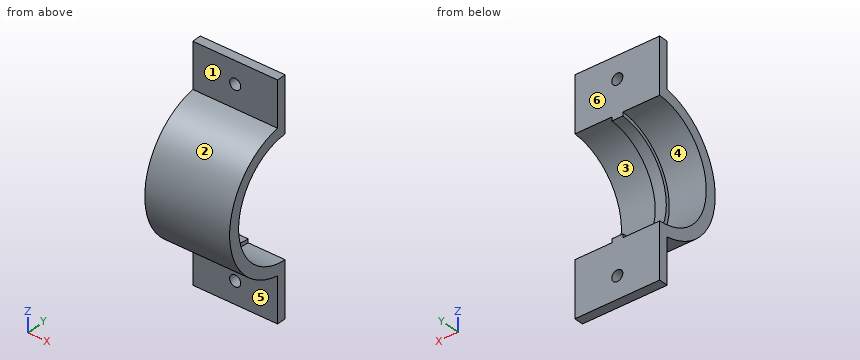
```python
from build123d import *

# Parameters (mm, degrees)
SKETCH3_W           = 13.566130208
SKETCH3_H           = 6
BOSS_EXTRUDE1_DEPTH = 11.5
SKETCH4_R           = 1.5
CUT_EXTRUDE1_DEPTH  = 11.5
SKETCH5_W           = 75.75040558
SKETCH5_H           = 1
CUT_EXTRUDE2_DEPTH  = 26


with BuildPart() as part:
    # Sketch2 → Revolve1 (revolve)
    with BuildSketch(Plane(origin=(0, 0, 0), x_dir=(1, 0, 0), z_dir=(0, 1, 0)), mode=Mode.PRIVATE) as revolve1_sk:
        Polygon((-11.5, 16), (-1.5, 16), (-1.5, 15), (1.5, 15), (1.5, 16), (11.5, 16), (11.5, 19), (-11.5, 19), align=None)
    revolve(revolve1_sk.sketch.rotate(Axis((-71.722155375, 0, 0), (1, 0, 0)), 180), axis=Axis((-71.722155375, 0, 0), (1, 0, 0)))

    # Sketch3 → Boss-Extrude1 (add, symmetric)
    with BuildSketch(Plane(origin=(0, 0, 0), x_dir=(0, 0, -1), z_dir=(1, 0, 0))):
        with Locations((24.243185686, 0)):
            Rectangle(SKETCH3_W, SKETCH3_H)
        with Locations((-24.243185686, 0)):
            Rectangle(SKETCH3_W, SKETCH3_H)
    extrude(amount=BOSS_EXTRUDE1_DEPTH, both=True)

    # Sketch4 → Cut-Extrude1 (cut, symmetric)
    with BuildSketch(Plane(origin=(0, 0, 0), x_dir=(1, 0, 0), z_dir=(0, 1, 0))):
        with Locations(Location((0, 25, 0), (0, 0, 270))):
            Circle(SKETCH4_R)
        with Locations(Location((0, -25, 0), (0, 0, 270))):
            Circle(SKETCH4_R)
    extrude(amount=CUT_EXTRUDE1_DEPTH, both=True, mode=Mode.SUBTRACT)

    # Sketch5 → Cut-Extrude2 (cut, symmetric)
    with BuildSketch(Plane(origin=(0, 0, 0), x_dir=(0, 0, -1), z_dir=(1, 0, 0))):
        Rectangle(SKETCH5_W, SKETCH5_H)
    extrude(amount=CUT_EXTRUDE2_DEPTH, both=True, mode=Mode.SUBTRACT)


with BuildPart() as cut_extrude2_piece_1:
    # of the separate pieces the step leaves, piece 1, a body of its own (cut_extrude2_pieces)
    add(part.part.solids().sort_by_distance((-11.5, 0.5, -15.992185592))[0])


with BuildPart() as cut_extrude2_piece_2:
    # of the separate pieces the step leaves, piece 2, a body of its own (cut_extrude2_pieces)
    add(part.part.solids().sort_by_distance((-11.5, -0.5, 15.992185592))[0])


solid = cut_extrude2_piece_2.part
```
Verification items for the finished model (mm, model axes). Face numbers are marked on the shaded views. A direction names the side the tool comes from. Round coordinates to 2 decimals unless told otherwise and drop trailing zeros. Order: outer loops, then holes, each group sorted by start corner. A loop starts at its lowest first (then second) coordinate and runs counter-clockwise, first axis right, second up. Notation, with made-up numbers: (45.5, 68.25) - (56.5, 68.25) arc R33 cw to (56.5, 100.25) - close; hole circle Ø10 at (-12.5, 67.5). An arc over 180 degrees is marked (long way). Use CSV: the item, a comma, the result in double quotes. Start each with the question number.
1) Mould release check, pull along Z, two halves, no side actions. Record for the marked faces 1, 2, 3 and 4: +Z half, -Z half, draft (parallel to the pull), parting line (faces both ways), or undercut.
2) Thickness scan on L1, parallel to X at y = -1.3, z = -25; L2, parallel to Y at x = 5.25, z = 21; L3, parallel to Z at x = 1.25, y = -4.5. Record the ranges inside material, lowest first.
3) Section check A-A, the plane z = 25. Record the cut outline in (x, y), plus the area to 3 significant figures.
4) Section check D-D, the plane z = 0. Record the cut outline in (x, y).
5) Section check B-B, the plane x = 0. Record the cut outline in (y, z).
6) Go/stop test with flat-tipped pins: P1, Ø12, axis at x = -6, z = -7, coming from the +Y side; P2, Ø2.5, axis at x = 0, z = -25, coming from the -Y side; P3, Ø1.5, axis at x = -5.5, z = 5, coming from the -Y side; P4, Ø3.5, axis at x = -3.5, z = -24.5, coming from the -Y side. Record where each tip stops, or that it passes through.
7) Section check C-C, the plane x = -8. Record the cut outline in (y, z), plus the area to 3 significant figures.
8) Access from +Z, -Z, +X, -X, +Y, -Y to the whole of each face (thin tool, end or side, straight path). Record for the marked faces 5 and 6.
Answers:
1,face 1,"draft"
1,face 2,"parting line"
1,face 3,"undercut"
1,face 4,"undercut"
2,L1,"x = -11.5 to -1.5, 1.5 to 11.5"
2,L2,"y = -3 to -0.5"
2,L3,"z = -18.46 to -14.31, 14.31 to 18.46"
3,outline,"(-11.5, -3) - (-1.5, -3) - (-1.5, -0.5) - (-11.5, -0.5) - close; (1.5, -3) - (11.5, -3) - (11.5, -0.5) - (1.5, -0.5) - close"
3,area,"50.0 mm²"
4,outline,"(-11.5, -19) - (11.5, -19) - (11.5, -16) - (1.5, -16) - (1.5, -15) - (-1.5, -15) - (-1.5, -16) - (-11.5, -16) - close"
5,outline,"(-3, -31.03) - (-0.5, -31.03) - (-0.5, -26.5) - (-3, -26.5) - close; (-3, -23.5) - (-0.5, -23.5) - (-0.5, -14.99) arc R15 cw to (-0.5, 14.99) - (-0.5, 23.5) - (-3, 23.5) - (-3, 18.76) arc R19 ccw to (-3, -18.76) - close; (-3, 26.5) - (-0.5, 26.5) - (-0.5, 31.03) - (-3, 31.03) - close"
6,P1,"stops at y = -9.33"
6,P2,"passes through"
6,P3,"stops at y = -18.52"
6,P4,"stops at y = -3"
7,outline,"(-3, -31.03) - (-0.5, -31.03) - (-0.5, -15.99) arc R16 cw to (-0.5, 15.99) - (-0.5, 31.03) - (-3, 31.03) - (-3, 18.76) arc R19 ccw to (-3, -18.76) - close"
7,area,"223 mm²"
8,face 5,"-Z, +X, -X, -Y"
8,face 6,"+Z, -Z, +X, -X, +Y"
